```python
from build123d import *

# Parameters (mm, degrees)
SKETCH1_R           = 30
BOSS_EXTRUDE1_DEPTH = 100
SHELL1_T            = -2
FILLET1_R           = 2
SKETCH2_R           = 10
BOSS_EXTRUDE2_DEPTH = 5
SKETCH3_R           = 2.5
CUT_EXTRUDE1_DEPTH  = 114.247516529


with BuildPart() as part:
    # Sketch1 → Boss-Extrude1 (new body)
    with BuildSketch(Plane.XY):
        Circle(SKETCH1_R)
    extrude(amount=BOSS_EXTRUDE1_DEPTH)

    # Shell1
    shell1_openings = [part.faces().sort_by_distance(p)[0] for p in [
        (0, 0, 100),
    ]]
    offset(amount=SHELL1_T, openings=shell1_openings, kind=Kind.INTERSECTION)

    # Fillet1
    fillet1_edges = [part.edges().sort_by_distance(p)[0] for p in [
        (-30, 0, 0),
    ]]
    fillet(fillet1_edges, radius=FILLET1_R)

    # Sketch2 → Boss-Extrude2 (add)
    with BuildSketch(Plane(origin=(0, 0, 0), x_dir=(-1, 0, 0), z_dir=(0, 0, -1))):
        with Locations(Location((0, 0, 0), (0, 0, 180))):
            Circle(SKETCH2_R)
    extrude(amount=BOSS_EXTRUDE2_DEPTH)

    # Sketch3 → Cut-Extrude1 (cut, through all)
    with BuildSketch(Plane(origin=(0, 0, -5), x_dir=(-1, 0, 0), z_dir=(0, 0, -1))):
        Circle(SKETCH3_R)
    extrude(amount=-CUT_EXTRUDE1_DEPTH, mode=Mode.SUBTRACT)


solid = part.part
```
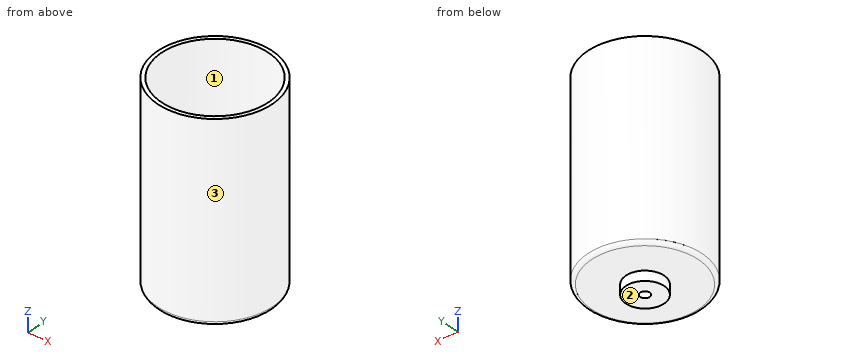
Geometry check sheet. Reference: the model listing, model coordinates, mm. Face numbers are marked on the shaded views. Coordinates: 2 decimals unless noted, no trailing zeros. Order: outer loops, then holes, each group sorted by start corner. A loop starts at its lowest first (then second) coordinate and runs counter-clockwise, first axis right, second up.
Item 1: Depth check by flat-ended pin: pin 1 (6 mm diameter, centred on x = 7.5, y = -9.5, fed in from +Z); pin 2 (12 mm diameter, centred on x = 15.5, z = 12.5, fed in from +Y); pin 3 (3 mm diameter, centred on x = -3.5, y = 23, fed in from -Z); pin 4 (4 mm diameter, centred on x = 0, y = 0, fed in from -Z). Enter the tip coordinate at first touch or a pass-through.
Item 2: Mould release check, pull along X, two halves, no side actions. Record for the marked faces 1, 2 and 3: released by +X, released by -X, zero draft, split by the parting line, or undercut.
Item 3: Scan lines: line 1 along Y through (x, z) = (0, 62.5); line 2 along Z through (x, y) = (1.5, -27); line 3 along Y through (x, z) = (0, -0.25). Record each from-to range of solid material in increasing order.
Item 4: Section check C-C (z = 57.5). Enter the section's corners in (x, y), plus the area to 3 significant figures.
Item 5: Section check A-A (x = 0). Enter the section's corners in (y, z).
Check sheet entries:
1. pin 1: stops at z = 2
1. pin 2: stops at y = 28.46
1. pin 3: stops at z = 0
1. pin 4: passes through
2. face 1: undercut
2. face 2: zero draft
2. face 3: split by the parting line
3. line 1: y = -30 to -28, 28 to 30
3. line 2: z = 0 to 2
3. line 3: y = -10 to -2.5, 2.5 to 10
4. outline: circle Ø60 at (0, 0); hole circle Ø56 at (0, 0)
4. area: 364 mm2
5. outline: (-30, 2) arc R2 ccw to (-28, 0) - (-10, 0) - (-10, -5) - (-2.5, -5) - (-2.5, 2) - (-28, 2) - (-28, 100) - (-30, 100) - close; (2.5, -5) - (10, -5) - (10, 0) - (28, 0) arc R2 ccw to (30, 2) - (30, 100) - (28, 100) - (28, 2) - (2.5, 2) - close
